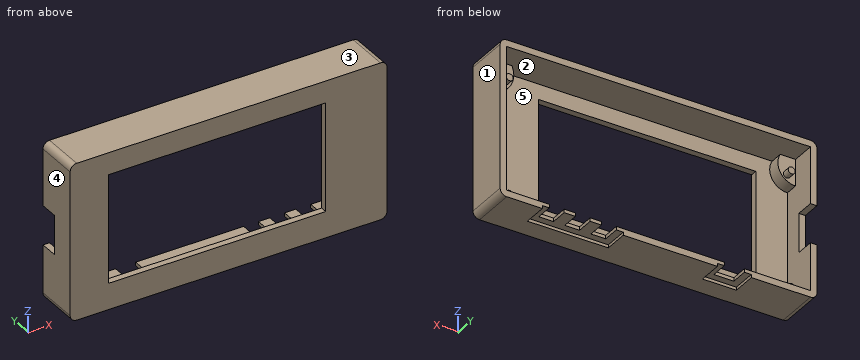
```python
from build123d import *

# Parameters (mm, degrees)
EXTRUDE_1_DEPTH         = 1.5
CUT_EXTRUDE_2_REACH     = 41.107
SKETCH_1_6_W            = 50
SKETCH_1_6_H            = 24.956
EXTRUDE_1_2_OUTLINE_W   = 72.855
EXTRUDE_1_2_OUTLINE_H   = 36.02
EXTRUDE_1_2_OUTLINE_W_2 = 69.855
EXTRUDE_1_2_OUTLINE_H_2 = 33.02
EXTRUDE_1_2_DEPTH       = 10
FILLET_1_R              = 1.5
EXTRUDE_2_DEPTH         = 3
SKETCH_3_R              = 0.8
EXTRUDE_3_DEPTH         = 1.8
CUT_EXTRUDE_3_REACH     = 76.522
SKETCH_4_W              = 9
SKETCH_4_H              = 4.3
CUT_EXTRUDE_4_REACH     = 53.172
SKETCH_5_W              = 3.4
SKETCH_5_H              = 4
SKETCH_5_W_2            = 4.6
CUT_EXTRUDE_START       = -1.5
SKETCH_5_6_W            = 7.8
SKETCH_5_6_H            = 7.2
SKETCH_5_6_W_2          = 18.6
CUT_EXTRUDE_6_DEPTH     = 0.7


# Read off the part's stored shape, not the designer's step: the extrude step
with BuildPart() as part:
    # Sketch 1 → Extrude 1 (new body)
    with BuildSketch(Plane(origin=(0, 0, 0), x_dir=(1, 0, 0), z_dir=(0, 1, 0))):
        Polygon((-34.9275, 15.494), (34.9275, 15.494), (34.9275, -15.494), (34.9275, -17.526), (-34.9275, -17.526), (-34.9275, -15.494), align=None)
    extrude(amount=EXTRUDE_1_DEPTH)

    # Sketch 1_6 → Cut-Extrude 2 (cut, up to next)
    with BuildSketch(Plane(origin=(0, 0, 0), x_dir=(1, 0, 0), z_dir=(0, 1, 0)), mode=Mode.PRIVATE) as cut_extrude_2_sk1:
        with Locations((-2.6635, -1.516)):
            Rectangle(SKETCH_1_6_W, SKETCH_1_6_H)
    cut_extrude_2_tool1 = extrude(cut_extrude_2_sk1.sketch, amount=CUT_EXTRUDE_2_REACH, mode=Mode.PRIVATE) & part.part
    add(cut_extrude_2_tool1.solids().sort_by_distance((-2.6635, 0, 1.516))[0], mode=Mode.SUBTRACT)



with BuildPart() as body_2:
    # Extrude 1 2 outline → Extrude 1 2 (new body)
    with BuildSketch(Plane(origin=(0, 0, 0), x_dir=(1, 0, 0), z_dir=(0, 1, 0))):
        with Locations((0, -1.016)):
            Rectangle(EXTRUDE_1_2_OUTLINE_W, EXTRUDE_1_2_OUTLINE_H)
        with Locations((0, -1.016)):
            Rectangle(EXTRUDE_1_2_OUTLINE_W_2, EXTRUDE_1_2_OUTLINE_H_2, mode=Mode.SUBTRACT)
    extrude(amount=EXTRUDE_1_2_DEPTH)

    # Fillet 1
    fillet_1_edges = [body_2.edges().sort_by_distance(p)[0] for p in [
        (-36.4275, 5, -16.994),
        (-36.4275, 5, 19.026),
        (36.4275, 5, 19.026),
        (36.4275, 5, -16.994),
    ]]
    fillet(fillet_1_edges, radius=FILLET_1_R)


with BuildPart() as part_1:
    add(part.part)

    add(body_2.part)  # Extrude 2 merges body 2
    # Sketch 2 → Extrude 2 (add)
    with BuildSketch(Plane(origin=(0, 1.5, 0), x_dir=(1, 0, 0), z_dir=(0, 1, 0))):
        with BuildLine():
            ThreePointArc((-31.407972759, -17.526), (-31.407972759, -13.462), (-34.9275, -11.43))
            Line((-34.9275, -11.43), (-34.9275, -17.526))
            Line((-34.9275, -17.526), (-31.407972759, -17.526))
        make_face()
        with BuildLine():
            ThreePointArc((-34.9275, 11.43), (-32.053818041, 12.620318041), (-30.8635, 15.494))
            Line((-30.8635, 15.494), (-34.9275, 15.494))
            Line((-34.9275, 15.494), (-34.9275, 11.43))
        make_face()
        with BuildLine():
            Line((34.9275, 15.494), (29.8635, 15.494))
            ThreePointArc((29.8635, 15.494), (31.34671126, 11.91321126), (34.9275, 10.43))
            Line((34.9275, 10.43), (34.9275, 15.494))
        make_face()
        with BuildLine():
            Line((34.9275, -17.526), (34.9275, -10.43))
            ThreePointArc((34.9275, -10.43), (30.688741691, -12.723255696), (30.289065781, -17.526))
            Line((30.289065781, -17.526), (34.9275, -17.526))
        make_face()
    extrude(amount=EXTRUDE_2_DEPTH)

    # Sketch 3 → Extrude 3 (add)
    with BuildSketch(Plane(origin=(0, 4.5, 0), x_dir=(1, 0, 0), z_dir=(0, 1, 0))):
        with Locations(Location((-32.9275, -13.394, 0), (0, 0, 270))):
            Circle(SKETCH_3_R)
        with Locations(Location((-32.9275, 13.394, 0), (0, 0, 90))):
            Circle(SKETCH_3_R)
        with Locations(Location((31.9275, -13.394, 0), (0, 0, 90))):
            Circle(SKETCH_3_R)
        with Locations(Location((31.9275, 13.394, 0), (0, 0, 270))):
            Circle(SKETCH_3_R)
    extrude(amount=EXTRUDE_3_DEPTH)

    # Sketch 4 → Cut-Extrude 3 (cut, up to next)
    with BuildSketch(Plane(origin=(-34.9275, 0, 0), x_dir=(0, 0, -1), z_dir=(1, 0, 0)), mode=Mode.PRIVATE) as cut_extrude_3_sk1:
        with Locations((0, 7.85)):
            Rectangle(SKETCH_4_W, SKETCH_4_H)
    cut_extrude_3_tool1 = extrude(cut_extrude_3_sk1.sketch, amount=-CUT_EXTRUDE_3_REACH, mode=Mode.PRIVATE) & part_1.part
    add(cut_extrude_3_tool1.solids().sort_by_distance((-34.9275, 7.85, 0))[0], mode=Mode.SUBTRACT)

    # Sketch 5 → Cut-Extrude 4 (cut, up to next)
    with BuildSketch(Plane.XY.offset(-15.494), mode=Mode.PRIVATE) as cut_extrude_4_sk1:
        with Locations((11.4275, 8.1)):
            Rectangle(SKETCH_5_W, SKETCH_5_H)
    cut_extrude_4_tool1 = extrude(cut_extrude_4_sk1.sketch, amount=-CUT_EXTRUDE_4_REACH, mode=Mode.PRIVATE) & part_1.part
    # Sketch 5 → Cut-Extrude 4 (cut, up to next)
    with BuildSketch(Plane.XY.offset(-15.494), mode=Mode.PRIVATE) as cut_extrude_4_sk2:
        with Locations((17.4275, 8.1)):
            Rectangle(SKETCH_5_W, SKETCH_5_H)
    cut_extrude_4_tool2 = extrude(cut_extrude_4_sk2.sketch, amount=-CUT_EXTRUDE_4_REACH, mode=Mode.PRIVATE) & part_1.part
    # Sketch 5 → Cut-Extrude 4 (cut, up to next)
    with BuildSketch(Plane.XY.offset(-15.494), mode=Mode.PRIVATE) as cut_extrude_4_sk3:
        with Locations((23.4275, 8.1)):
            Rectangle(SKETCH_5_W, SKETCH_5_H)
    cut_extrude_4_tool3 = extrude(cut_extrude_4_sk3.sketch, amount=-CUT_EXTRUDE_4_REACH, mode=Mode.PRIVATE) & part_1.part
    # Sketch 5 → Cut-Extrude 4 (cut, up to next)
    with BuildSketch(Plane.XY.offset(-15.494), mode=Mode.PRIVATE) as cut_extrude_4_sk4:
        with Locations((-17.4275, 8.1)):
            Rectangle(SKETCH_5_W_2, SKETCH_5_H)
    cut_extrude_4_tool4 = extrude(cut_extrude_4_sk4.sketch, amount=-CUT_EXTRUDE_4_REACH, mode=Mode.PRIVATE) & part_1.part
    add(cut_extrude_4_tool1.solids().sort_by_distance((11.4275, 8.1, -15.494))[0], mode=Mode.SUBTRACT)
    add(cut_extrude_4_tool2.solids().sort_by_distance((17.4275, 8.1, -15.494))[0], mode=Mode.SUBTRACT)
    add(cut_extrude_4_tool3.solids().sort_by_distance((23.4275, 8.1, -15.494))[0], mode=Mode.SUBTRACT)
    add(cut_extrude_4_tool4.solids().sort_by_distance((-17.4275, 8.1, -15.494))[0], mode=Mode.SUBTRACT)

    # Sketch 5_6 → Cut-Extrude 6 (cut)
    with BuildSketch(Plane.XY.offset(-15.494).offset(CUT_EXTRUDE_START)):
        with Locations((-17.4275, 8.1)):
            Rectangle(SKETCH_5_6_W, SKETCH_5_6_H)
        with Locations((17.4275, 8.1)):
            Rectangle(SKETCH_5_6_W_2, SKETCH_5_6_H)
    extrude(amount=CUT_EXTRUDE_6_DEPTH, mode=Mode.SUBTRACT)


solid = part_1.part
```
CAD build for the part. Positions are in the model's coordinates, mm. Face numbers are marked on the shaded views. A direction names the side the tool comes from. Round coordinates to 2 decimals unless told otherwise and drop trailing zeros. Loops run counter-clockwise (first coordinate to the right, second up) from the corner with the lowest first, then second, coordinate; pieces in that order, holes last. Notation, with made-up numbers: M -36.75,11 L 4.25,11 A30 cw 4.25,47 Z; hole C 46,36 d4. An arc over 180 degrees is marked long. Use a Markdown table: item, result. Add a question column.
(1) Which spindle directions (+Z, -Z, +X, -X, +Y, -Y) get a long thin tool onto all of the face, cutting with end or side? Do the marked faces 1 and 2. Say none if no direction does.
(2) Flat gauge pins, fed straight in: pin 1 (0.6 mm diameter, centred on y = 8.5, z = -16, fed in from -X); pin 2 (0.6 mm diameter, centred on y = 9, z = -16, fed in from +X); pin 3 (0.6 mm diameter, centred on x = 12, z = -15.5, fed in from +Y); pin 4 (10 mm diameter, centred on x = 16.5, z = 8, fed in from -Y). Where does each tip first touch, or does it go through?
(3) Cut at D-D (x = 17.5). Give the cut face in (y, z), and give its area (3 significant figures).
(4) Cut at A-A (z = 5.5). Give the cut face in (x, y), and give its area (3 significant figures).
(5) Cut at C-C (z = 15.5). Give the cut face in (x, y).
(6) Cut at B-B (x = 1). Give the cut face in (y, z).
(7) Drill centre lines: line 1 (X direction, y = 7.5, z = 16); line 2 (X direction, y = 1.25, z = -1.5); line 3 (Z direction, x = 21, y = 9.75). Where is each one in solid material? Low to high.
(8) Pull direction X, two halves, no side cores. Call the marked faces 3, 4 and 5: +X half, -X half, draft (parallel to the pull), parting line (faces both ways), or undercut.
Geometry says:
| question | item | result |
|---|---|---|
| 1 | face 1 | +Z, -Z, +X, +Y, -Y |
| 1 | face 2 | +Y |
| 2 | pin 1 | stops at x = -36.41 |
| 2 | pin 2 | stops at x = 36.41 |
| 2 | pin 3 | stops at y = 6.1 |
| 2 | pin 4 | passes through |
| 3 | outline | M 0,-16.99 L 4.5,-16.99 L 4.5,-16.29 L 6.1,-16.29 L 6.1,-15.49 L 1.5,-15.49 L 1.5,-10.96 L 0,-10.96 Z; M 0,13.99 L 1.5,13.99 L 1.5,17.53 L 10,17.53 L 10,19.03 L 0,19.03 Z |
| 3 | area | 35.1 mm² |
| 4 | outline | M -36.43,0 L -27.66,0 L -27.66,1.5 L -34.93,1.5 L -34.93,10 L -36.43,10 Z; M 22.34,0 L 36.43,0 L 36.43,10 L 34.93,10 L 34.93,1.5 L 22.34,1.5 Z |
| 4 | area | 59.8 mm² |
| 5 | outline | M -36.43,0 L 36.43,0 L 36.43,10 L 34.93,10 L 34.93,4.5 L 29.86,4.5 L 29.86,1.5 L -30.86,1.5 L -30.86,4.5 L -34.93,4.5 L -34.93,10 L -36.43,10 Z |
| 6 | outline | M 0,-16.99 L 10,-16.99 L 10,-15.49 L 1.5,-15.49 L 1.5,-10.96 L 0,-10.96 Z; M 0,13.99 L 1.5,13.99 L 1.5,17.53 L 10,17.53 L 10,19.03 L 0,19.03 Z |
| 7 | line 1 | x = -36.43 to -34.93, 34.93 to 36.43 |
| 7 | line 2 | x = -36.43 to -27.66, 22.34 to 36.43 |
| 7 | line 3 | z = -16.29 to -15.49, 17.53 to 19.03 |
| 8 | face 3 | draft |
| 8 | face 4 | -X half |
| 8 | face 5 | undercut |
